Could you check a few things on this model? Use its own coordinates, in mm. A direction names the side the tool comes from. Give positions to 0.01 mm unless a question says otherwise; leave off trailing zeros. Loops run counter-clockwise (first coordinate to the right, second up) from the corner with the lowest first, then second, coordinate; pieces in that order, holes last. Notation, with made-up numbers: (0, 1) - (10, 1) arc R34 ccw to (10, 37) - close; hole circle Ø4 at (35.5, -6). An arc over 180 degrees is marked (long way). Write each question's results on one line, items separated by ' | '. Start each with the question number.
1) On a 3-axis mill with a long thin cutter (end or side, diameter ignored), from which of +Z, -Z, +X, -X, +Y, -Y can I reach the whole of each face in a straight line? I mean faces 1 (the face through (-31, 21, 0)), 2 (the face through (-31.58, 39.49, -2.85)), 3 (the face through (-31.58, 2.85, -3.01)). Say none if no direction works.
2) I want a section at B-B, the plane z = 10.5. Write out the boundary of the cut face in (x, y), and give its area (3 significant figures).
3) I'm going to push flat-ended pins straight in: pin 1 (11 mm diameter, centred on x = -24.5, y = 18.5, fed in from +Z); pin 2 (9 mm diameter, centred on y = 22, z = 12, fed in from -X). Where does each tip first touch, or does it pass through?
4) I want a section at C-C, the plane y = 13. Write out the boundary of the cut face in (x, z), and give its area (3 significant figures).
5) I want a section at A-A, the plane x = -40.5. Write out the boundary of the cut face in (y, z), and give its area (3 significant figures).
6) If I drill on probe 1 along X at (y, z) = (23, 11); probe 2 along Z at (x, y) = (-36, 17); probe 3 along Z at (x, y) = (-25, 2.5), over which ranges is the centre line in solid material (lowest first)? Write a range as [from, to].
Autodesk Inventor part; units mm, degrees
ref_plane "YZ Plane" through (0, 0, 0) normal (1, 0, 0) x (0, 1, 0)
ref_plane "XZ Plane" through (0, 0, 0) normal (0, 1, 0) x (-1, 0, 0)
ref_plane "XY Plane" through (0, 0, 0) normal (0, 0, 1) x (1, 0, 0)
sketch "Sketch1" plane through (0, 0, 0) normal (0, 1, 0) x (-1, 0, 0)
  line L0 (14.6941, 0) -> (51, 0)
  line L1 (51, 0) -> (51, -146)
  line L2 (51, -146) -> (0, -146)
  line L3 (0, -146) -> (0, 0)
  line L4 (14.6941, 0) -> (14.6941, 20.4717)
  line L5 (14.6941, 20.4717) -> (0, 20.4717)
  line L6 (0, 20.4717) -> (0, 0)
  dimension "d0" = 51
  dimension "d1" = 146
extrude "Extrusion1" add sketch "Sketch1" along normal blind 42.5
fillet "Fillet1" radius 10 2 edges at (-32.847, 42.5, 0) (-32.847, 0, 0)
fillet "Fillet2" radius 3 11 edges at (-51, 2.9289, -2.9289) (-51, 21.25, 0) (-51, 39.5711, -2.9289) (-51, 42.5, -78) (-51, 0, -78) (-51, 21.25, -146) (-25.5, 0, -146) (0, 21.25, -146) (0, 0, -73) (0, 42.5, -73) (-25.5, 42.5, -146)
properties part number "Flight Battery 5000 mah 5S"
Answers:
1) face 1: +Z, -X, +Y, -Y | face 2: +Z, -X, +Y | face 3: +Z, -X, -Y
2) outline: (-14.69, 0) - (-3, 0) arc R3 ccw to (0, 3) - (0, 39.5) arc R3 ccw to (-3, 42.5) - (-14.69, 42.5) - close | area: 621 mm2
3) pin 1: stops at z = 0 | pin 2: stops at x = -14.69
4) outline: (-51, -143) arc R3 ccw to (-48, -146) - (-3, -146) arc R3 ccw to (0, -143) - (0, 20.47) - (-14.69, 20.47) - (-14.69, 0) - (-48, 0) arc R3 ccw to (-51, -3) - close | area: 7,740 mm2
5) outline: (0, -143) arc R3 ccw to (3, -146) - (39.5, -146) arc R3 ccw to (42.5, -143) - (42.5, -10) arc R10 ccw to (32.5, 0) - (10, 0) arc R10 ccw to (0, -10) - close | area: 6,160 mm2
6) probe 1: x = [-14.69, 0] | probe 2: z = [-146, 0] | probe 3: z = [-145.96, -3.39]
